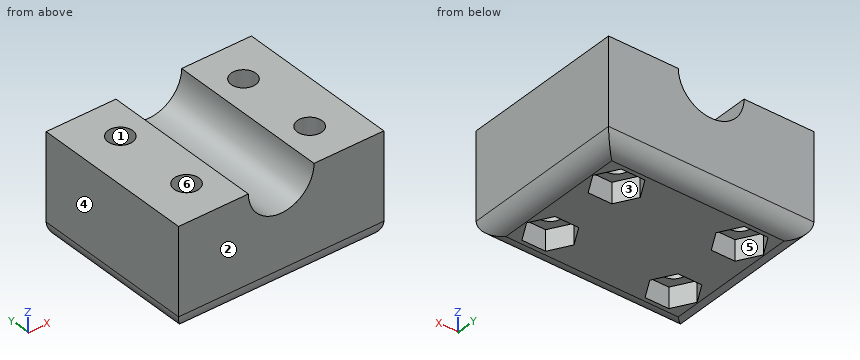
```python
from build123d import *

# Parameters (mm, degrees)
SKETCH1_W           = 50
SKETCH1_H           = 40
BOSS_EXTRUDE1_DEPTH = 25
SKETCH2_R           = 8
CUT_EXTRUDE1_DEPTH  = 43
SKETCH3_R           = 3
CUT_EXTRUDE2_DEPTH  = 43
CUT_EXTRUDE3_DEPTH  = 5
FILLET1_R           = 4


with BuildPart() as part:
    # Sketch1 → Boss-Extrude1 (new body)
    with BuildSketch(Plane.XY):
        with Locations((25, 20)):
            Rectangle(SKETCH1_W, SKETCH1_H)
    extrude(amount=BOSS_EXTRUDE1_DEPTH)

    # Sketch2 → Cut-Extrude1 (cut)
    with BuildSketch(Plane(origin=(0, 40, 0), x_dir=(1, 0, 0), z_dir=(0, 1, 0))):
        with Locations((25, -25)):
            Circle(SKETCH2_R)
    extrude(amount=-CUT_EXTRUDE1_DEPTH, mode=Mode.SUBTRACT)

    # Sketch3 → Cut-Extrude2 (cut)
    with BuildSketch(Plane.XY.offset(25)):
        with Locations((10, 30)):
            Circle(SKETCH3_R)
        with Locations((10, 10)):
            Circle(SKETCH3_R)
        with Locations((40, 30)):
            Circle(SKETCH3_R)
        with Locations((40, 10)):
            Circle(SKETCH3_R)
    extrude(amount=-CUT_EXTRUDE2_DEPTH, mode=Mode.SUBTRACT)

    # Sketch4 → Cut-Extrude3 (cut)
    with BuildSketch(Plane(origin=(0, 0, 0), x_dir=(-1, 0, 0), z_dir=(0, 0, -1))):
        Polygon((-7.113248654, 5), (-4.226497308, 10), (-7.113248654, 15), (-12.886751346, 15), (-15.773502692, 10), (-12.886751346, 5), align=None)
        Polygon((-37.113248654, 5), (-34.226497308, 10), (-37.113248654, 15), (-42.886751346, 15), (-45.773502692, 10), (-42.886751346, 5), align=None)
        Polygon((-7.113248654, 25), (-4.226497308, 30), (-7.113248654, 35), (-12.886751346, 35), (-15.773502692, 30), (-12.886751346, 25), align=None)
        Polygon((-42.886751346, 35), (-45.773502692, 30), (-42.886751346, 25), (-37.113248654, 25), (-34.226497308, 30), (-37.113248654, 35), align=None)
    extrude(amount=-CUT_EXTRUDE3_DEPTH, mode=Mode.SUBTRACT)

    # Fillet1
    fillet1_edges = [part.edges().sort_by_distance(p)[0] for p in [
        (25, 40, 0),
        (50, 20, 0),
        (25, 0, 0),
        (0, 20, 0),
    ]]
    fillet(fillet1_edges, radius=FILLET1_R)


solid = part.part
```
The listing builds one solid part. Answer for the finished solid, in the listing's coordinates (mm). Face numbers are marked on the shaded views. A direction names the side the tool comes from. Coordinates: 2 decimals unless noted, no trailing zeros. Loops run counter-clockwise (first coordinate to the right, second up) from the corner with the lowest first, then second, coordinate; pieces in that order, holes last. Notation, with made-up numbers: (23, 33) - (47, 33) arc R26 ccw to (47, 67) - close; hole circle Ø8 at (26.5, 20.25). An arc over 180 degrees is marked (long way). Use a Markdown table: item, result. Add a question column.
1) Find the intervals of material crossed by line 1 (Y direction, x = 7.5, z = 3.75); line 2 (Y direction, x = 40, z = 12); line 3 (X direction, y = 36, z = 21.5), in increasing order.
2) The part is cut by section B-B, the plane x = 10. Give the vertices of the cut face in (y, z).
3) Given pin 1 (1.5 mm diameter, centred on x = 10, z = 1.5, fed in from -Y); pin 2 (2.5 mm diameter, centred on x = 11, z = 2, fed in from +Y); pin 3 (8 mm diameter, centred on x = 40, y = 30, fed in from -Z), each flat-ended and moving along its own axis, determine where each tip first touches the part or whether it passes through.
4) For the marked faces 5 and 6, determine the directions among +Z, -Z, +X, -X, +Y, -Y from which every point of the face is accessible in a straight line to the end or side of a thin tool.
5) The part is cut by section C-C, the plane y = 11.5. Give the vertices of the cut face in (x, z), and give its area (3 significant figures).
6) The mould has two halves that part along X. Classify the marked faces 1, 2, 3 and 4: released by +X, released by -X, zero draft, split by the parting line, or undercut.
7) The part is cut by section A-A, the plane z = 14.75. Give the vertices of the cut face in (x, y), and give its area (3 significant figures).
8) The part is cut by section D-D, the plane y = 21. Give the vertices of the cut face in (x, z).
Here are the results:
| question | item | result |
|---|---|---|
| 1 | line 1 | y = 0.01 to 5, 15 to 25, 35 to 39.99 |
| 1 | line 2 | y = 0 to 7, 13 to 27, 33 to 40 |
| 1 | line 3 | x = 0 to 17.81, 32.19 to 50 |
| 2 | outline | (0, 4) arc R4 ccw to (4, 0) - (5, 0) - (5, 5) - (7, 5) - (7, 25) - (0, 25) - close; (13, 5) - (15, 5) - (15, 0) - (25, 0) - (25, 5) - (27, 5) - (27, 25) - (13, 25) - close; (33, 5) - (35, 5) - (35, 0) - (36, 0) arc R4 ccw to (40, 4) - (40, 25) - (33, 25) - close |
| 3 | pin 1 | stops at y = 0.4 |
| 3 | pin 2 | stops at y = 39.93 |
| 3 | pin 3 | stops at z = 5 |
| 4 | face 5 | -Z |
| 4 | face 6 | +Z, -Z |
| 5 | outline | (0, 4) arc R4 ccw to (4, 0) - (5.09, 0) - (5.09, 5) - (7.4, 5) - (7.4, 25) - (0, 25) - close; (12.6, 5) - (14.91, 5) - (14.91, 0) - (35.09, 0) - (35.09, 5) - (37.4, 5) - (37.4, 25) - (33, 25) arc R8 cw to (17, 25) - (12.6, 25) - close; (42.6, 5) - (44.91, 5) - (44.91, 0) - (46, 0) arc R4 ccw to (50, 4) - (50, 25) - (42.6, 25) - close |
| 5 | area | 837 mm^2 |
| 6 | face 1 | undercut |
| 6 | face 2 | zero draft |
| 6 | face 3 | undercut |
| 6 | face 4 | released by -X |
| 7 | outline | (0, 0) - (50, 0) - (50, 40) - (0, 40) - close; hole circle Ø6 at (10, 10); hole circle Ø6 at (10, 30); hole circle Ø6 at (40, 10); hole circle Ø6 at (40, 30) |
| 7 | area | 1,890 mm^2 |
| 8 | outline | (0, 4) arc R4 ccw to (4, 0) - (46, 0) arc R4 ccw to (50, 4) - (50, 25) - (33, 25) arc R8 cw to (17, 25) - (0, 25) - close |
